Check sheet for the modelled part. Datum: model origin and axes. Units: mm. A direction names the side the tool comes from. Round coordinates to 2 decimals unless told otherwise and drop trailing zeros. Loops run counter-clockwise (first coordinate to the right, second up) from the corner with the lowest first, then second, coordinate; pieces in that order, holes last. Notation, with made-up numbers: (26, 33) -> (44, 33) arc R28 cw to (44, 72) -> close; hole circle Ø9 at (53.5, 14.5). An arc over 180 degrees is marked (long way). Use one line per item in the form item = value. Start each with the question number.
(1) Material ranges on probe 1 along Y at (x, z) = (0, 7); probe 2 along Z at (x, y) = (6.5, -0.5); probe 3 along Y at (x, z) = (1.25, 10.75), recorded low to high. Write a range as [from, to].
(2) Go/stop test with flat-tipped pins: pin 1 (4 mm diameter, centred on y = 4, z = 9.5, fed in from +X); pin 2 (5.5 mm diameter, centred on x = 0.5, z = 8.5, fed in from +Y); pin 3 (3.5 mm diameter, centred on x = -0.5, z = 6.5, fed in from -Y). Record where each tip stops, or that it passes through.
(3) Sectioned sample at D-D (z = 4.5). Record the cut outline in (x, y), and give its area (3 significant figures).
(4) Sectioned sample at A-A (x = 0). Record the cut outline in (y, z), and give its area (3 significant figures).
(5) Sectioned sample at C-C (z = 1.75). Record the cut outline in (x, y), and give its area (3 significant figures).
(6) Set-up check for faces 1 (the cylindrical face through (-3.2, -2.4, 5.9)), 2 (the flat face through (-0.1, -4.2, 10)), 3 (the flat face through (0, -2.104, 8)): record each of +Z, -Z, +X, -X, +Y, -Y from which the full face is reachable in a straight line by a thin tool's end or side.
(7) Draft check along Z on faces 4 (the flat face through (0, 2.104, 8)), 5 (the flat face through (0, 3, 11)), 6 (the flat face through (0, 0, 0)), 7 (the flat face through (-0.1, 4.2, 10)). Enter one of: released by +Z, released by -Z, zero draft, split by the parting line, or undercut.
from build123d import *

# Parameters (mm, degrees)
SKETCH1_R               = 8
BOSS_EXTRUDE1_DEPTH     = 2
SKETCH2_R               = 4
BOSS_EXTRUDE2_DEPTH     = 9
SKETCH7_R               = 5
CUT_EXTRUDE1_DEPTH      = 9
CUT_EXTRUDE1_DEPTH_BACK = 9


with BuildPart() as part:
    # Sketch1 → Boss-Extrude1 (new body)
    with BuildSketch(Plane.XY):
        Circle(SKETCH1_R)
    extrude(amount=BOSS_EXTRUDE1_DEPTH)

    # Sketch2 → Boss-Extrude2 (add)
    with BuildSketch(Plane.XY.offset(2)):
        Circle(SKETCH2_R)
    extrude(amount=BOSS_EXTRUDE2_DEPTH)

    # Sketch7 → section 0 of loft1
    with BuildSketch(Plane.XY.offset(10), mode=Mode.PRIVATE) as loft1_s0:
        Circle(SKETCH7_R)
    # loft up to a face of the part (loft1)
    loft([loft1_s0.sketch, part.faces().sort_by_distance((0, 0, 11))[0]])

    # Sketch4 → Cut-Extrude1 (cut, two sides: drawn at the far end of the back side and taken through both)
    with BuildSketch(Plane(origin=(0, 0, 0), x_dir=(0, 0, -1), z_dir=(1, 0, 0)).offset(-CUT_EXTRUDE1_DEPTH_BACK)):
        with BuildLine():
            Line((-11, 2.103629109), (-4.141860423, 2.103629109))
            ThreePointArc((-4.141860423, 2.103629109), (-2.038231313, 0), (-4.141860423, -2.103629109))
            Line((-4.141860423, -2.103629109), (-11, -2.103629109))
            ThreePointArc((-11, -2.103629109), (-13.103629109, 0), (-11, 2.103629109))
        make_face()
    extrude(amount=CUT_EXTRUDE1_DEPTH + CUT_EXTRUDE1_DEPTH_BACK, mode=Mode.SUBTRACT)


solid = part.part
Checks:
q1.probe_1 = [-4, -2.1], [2.1, 4]
q1.probe_2 = [0, 2]
q1.probe_3 = [-4.06, -2.1], [2.1, 4.06]
q2.pin_1 = 4.54
q2.pin_2 = 5
q2.pin_3 = -4
q3.outline = (-3.4, -2.1) arc R4 ccw to (3.4, -2.1) -> close; (-3.4, 2.1) -> (3.4, 2.1) arc R4 ccw to start
q3.area = 18.2 mm2
q4.outline = (-8, 0) -> (8, 0) -> (8, 2) -> (4, 2) -> (4, 10) -> (5, 10) -> (4, 11) -> (2.1, 11) -> (2.1, 4.14) arc R2.1 cw to (-2.1, 4.14) -> (-2.1, 11) -> (-4, 11) -> (-5, 10) -> (-4, 10) -> (-4, 2) -> (-8, 2) -> close
q4.area = 69.2 mm2
q5.outline = circle Ø16 at (0, 0)
q5.area = 201 mm2
q6.face_1 = none
q6.face_2 = -Y
q6.face_3 = +Z, +X, -X
q7.face_4 = zero draft
q7.face_5 = released by +Z
q7.face_6 = released by -Z
q7.face_7 = undercut
